The model under review builds one solid part; all positions refer to its coordinate system, in mm. A direction names the side the tool comes from. Coordinates: 2 decimals unless noted, no trailing zeros. Order: outer loops, then holes, each group sorted by start corner. A loop starts at its lowest first (then second) coordinate and runs counter-clockwise, first axis right, second up. Notation, with made-up numbers: M -3.75,82.5 L 26.25,82.5 A15 cw 26.25,86.5 Z; hole C -11,-18.5 d2. An arc over 180 degrees is marked long. Write each question's results on one line, items separated by ' | '.
from build123d import *

# Parameters (mm, degrees)
F0_W     = 27.305
F0_H     = 55.88
F1_DEPTH = 101.6
F2_R     = 8.3312
F3_DEPTH = 38.1
F4_R     = 12.7
F4_R_2   = 8.3312
F5_DEPTH = 12.7


with BuildPart() as f1:
    # F0 (on Front) → F1 (new body, symmetric)
    with BuildSketch(Plane.XZ):
        with Locations((13.6525, 27.94)):
            Rectangle(F0_W, F0_H)
    extrude(amount=F1_DEPTH, both=True)

    # F2 (on face) → F3 (cut)
    with BuildSketch(Plane.YZ.offset(27.305)):
        with Locations((-60.325, 30.988)):
            Circle(F2_R)
        with Locations((60.325, 30.988)):
            Circle(F2_R)
    extrude(amount=-F3_DEPTH, mode=Mode.SUBTRACT)

    # F4 (on face) → F5 (cut)
    with BuildSketch(Plane.YZ.offset(27.305)):
        with Locations((-60.325, 30.988)):
            Circle(F4_R)
        with Locations((-60.325, 30.988)):
            Circle(F4_R_2, mode=Mode.SUBTRACT)
        with Locations((60.325, 30.988)):
            Circle(F4_R)
        with Locations((60.325, 30.988)):
            Circle(F4_R_2, mode=Mode.SUBTRACT)
    extrude(amount=-F5_DEPTH, mode=Mode.SUBTRACT)


solid = f1.part
1) Take a section at C-C on x = 5.5. State the section outline as (y, z) points (3 decimals).
Solutions:
outline: M -101.6,0 L 101.6,0 L 101.6,55.88 L -101.6,55.88 Z; hole C -60.325,30.988 d16.662; hole C 60.325,30.988 d16.662
2) For faces 1 (the cylindrical face through (21.044, 50.247, 23.26)), 2 (the flat face through (13, -1, 55.88)), list the 3-axis set-ups (+Z, -Z, +X, -X, +Y, -Y) from which the entire face can be reached by the end or side of a thin tool; tool diameter is ignored.
Solutions:
face 1: +X | face 2: +Z, +X, -X, +Y, -Y
3) The part is to be moulded in two halves that separate along Z. For faces 3 (the cylindrical face through (21.044, -54.465, 19.721)), 4 (the flat face through (13, -1, 0)), 5 (the flat face through (27.305, -1, 28)), say which applies: pulls with the +Z half, pulls with the -Z half, needs draft (parallel to the pull), parting line crosses it, or undercut.
Solutions:
face 3: undercut | face 4: pulls with the -Z half | face 5: needs draft
4) Take a section at B-B on x = 25.5. State the section outline as (y, z) points (3 decimals), plus the area to 3 significant figures.
Solutions:
outline: M -101.6,0 L 101.6,0 L 101.6,55.88 L -101.6,55.88 Z; hole C -60.325,30.988 d25.4; hole C 60.325,30.988 d25.4 | area: 10,300 mm2
5) To check wall thickness, follow line 1 along Y through (x, z) = (20, 30); line 2 along Y through (x, z) = (20.75, 35); line 3 along Z through (x, y) = (20.75, 67). State the ranges of each line that lie inside material, in increasing order.
Solutions:
line 1: -101.6 to -72.99, -47.66 to 47.66, 72.99 to 101.6 | line 2: -101.6 to -72.37, -48.28 to 48.28, 72.37 to 101.6 | line 3: 0 to 20.18, 41.79 to 55.88
6) For pin 1 (10 mm diameter, centred on x = 14.5, y = -53.5, fed in from -Z); pin 2 (20.5 mm diameter, centred on y = 60.325, z = 30.988, fed in from +X) (3 decimals); pin 3 (15 mm diameter, centred on y = -60.325, z = 30.988, fed in from -X) (3 decimals), all flat-tipped, find the tip position at first contact; note any pin that passes through.
Solutions:
pin 1: z = 0 | pin 2: x = 14.605 | pin 3: through
7) Take a section at A-A on y = -62.5. State the section outline as (x, z) points (3 decimals).
Solutions:
outline: M 0,0 L 27.305,0 L 27.305,18.476 L 14.605,18.476 L 14.605,22.946 L 0,22.946 Z; M 0,39.03 L 14.605,39.03 L 14.605,43.5 L 27.305,43.5 L 27.305,55.88 L 0,55.88 Z
